For this review, take the finished solid that the model builds, in its own axes (mm). A direction names the side the tool comes from. Coordinates: 2 decimals unless noted, no trailing zeros. Loops run counter-clockwise (first coordinate to the right, second up) from the corner with the lowest first, then second, coordinate; pieces in that order, holes last. Notation, with made-up numbers: (71, 69.5) -> (98, 69.5) arc R27 cw to (98, 85.5) -> close; hole circle Ø10 at (-32, 47.25). An arc over 180 degrees is marked (long way). Use a Markdown table: item, result.
Autodesk Inventor part; units mm, degrees
ref_plane "Work Plane1" through (3.5, 0, 0) normal (1, 0, 0) x (0, 1, 0)
ref_plane "XZ Plane" through (0, 0, 0) normal (0, 1, 0) x (-1, 0, 0)
ref_plane "XY Plane" through (0, 0, 0) normal (0, 0, 1) x (1, 0, 0)
sketch "Sketch1" plane through (0, 0, 0) normal (0, 1, 0) x (-1, 0, 0)
  circle A0 centre (0, 0) radius 2.2
  circle A1 centre (0, 0) radius 4.5
  dimension "d0" = 4.4
  dimension "d1" = 9
extrude "Extrusion1" add sketch "Sketch1" along normal blind 15 contours A0 | A1
sketch "Sketch2" plane through (0, 15, 0) normal (0, 1, 0) x (1, 0, 0)
  circle A0 centre (0, 0) radius 2.2
  dimension "d4" = 4.4
ref_plane "Work Plane1" through (3.5, 0, 0) normal (1, 0, 0) x (0, 1, 0)
sketch "Sketch3" plane through (3.5, 0, 0) normal (1, 0, 0) x (0, 1, 0)
  line L0 (0, 0) -> (7.5, 0)
  circle A0 centre (7.5, 0) radius 5.5
  dimension "d13" = 7.5
  dimension "d15" = 11
extrude "Extrusion2" add sketch "Sketch3" along normal mid plane 30
sketch "Sketch6" plane through (-11.5, 0, 0) normal (-1, 0, 0) x (0, 0, 1)
  circle A0 centre (0, 7.5) radius 5.5
  arc A1 (0, 11) -> (0, 4) centre (0, 7.5) ccw
  line L0 (0, 2) -> (0, 13)
  line L1 (0, 11) -> (0, 4)
  point P0 (0, 0)
sketch "Sketch7" plane through (18.5, 7.5, 0) normal (1, 0, 0) x (0, 0, -1)
  point P0 (0, -7.5)
hole "Hole4" at (0, 15, 0) direction (0, -1, 0) diameter 4.5 depth 20
sketch "Sketch8" plane through (18.5, 7.5, 0) normal (1, 0, 0) x (0, 0, -1)
  circle A0 centre (0, 0) radius 3
  point P0 (0, -7.5)
  dimension "d44" = 6
hole "Hole5" at (18.5, 7.5, 0) direction (-1, 0, 0) diameter 6 depth 15
properties part number "codo"
(1) Mouldability with a two-part tool opening along Y and no side actions: class faces 1 (the face through (-2, 15, -2)), 2 (the face through (10.895, 4.526, 0.391)), 3 (the face through (3.5, 7, 0)), 4 (the face through (18.5, 10, -2)) as pulls with the +Y half, pulls with the -Y half, needs draft (parallel to the pull), parting line crosses it, or undercut.
Found:
| item | result |
|---|---|
| face 1 | pulls with the +Y half |
| face 2 | undercut |
| face 3 | undercut |
| face 4 | needs draft |
(2) Take a section at C-C on y = 7.5. Write out the cut boundary in (x, z).
Found:
| item | result |
|---|---|
| outline | (-11.5, -5.5) -> (18.5, -5.5) -> (18.5, -3) -> (3.5, -3) -> (3.5, 3) -> (18.5, 3) -> (18.5, 5.5) -> (-11.5, 5.5) -> close; hole circle Ø4.5 at (0, 0) |
(3) For faces 5 (the face through (3.71, 6.784, 5.453)), 6 (the face through (0.98, 13.28, 4.39)), 7 (the face through (-2.08, 1.66, 3.99)), list the 3-axis set-ups (+Z, -Z, +X, -X, +Y, -Y) from which the entire face can be reached by the end or side of a thin tool; tool diameter is ignored.
Found:
| item | result |
|---|---|
| face 5 | none |
| face 6 | +Y |
| face 7 | -Y |
(4) Take a section at D-D on x = -9.5. Write out the cut boundary in (y, z).
Found:
| item | result |
|---|---|
| outline | circle Ø11 at (7.5, 0) |
(5) Take a section at A-A on z = 0. Write out the cut boundary in (x, y), plus the area to 4 significant figures.
Found:
| item | result |
|---|---|
| outline | (-11.5, 2) -> (-4.5, 2) -> (-4.5, 0) -> (-2.25, 0) -> (-2.25, 15) -> (-4.5, 15) -> (-4.5, 13) -> (-11.5, 13) -> close; (2.25, 0) -> (4.5, 0) -> (4.5, 2) -> (18.5, 2) -> (18.5, 4.5) -> (3.5, 4.5) -> (3.5, 10.5) -> (18.5, 10.5) -> (18.5, 13) -> (4.5, 13) -> (4.5, 15) -> (2.25, 15) -> close |
| area | 208.5 mm^2 |
(6) For pin 1 Ø2 at (x, z) = (-8.5, 2.5) entering from -Y; pin 2 Ø1.5 at (x, y) = (-3, 1.5) entering from +Z; pin 3 Ø4 at (x, z) = (-1, 0) entering from -Y; pin 4 Ø2 at (x, z) = (7, 2.5) entering from +Y, all flat-tipped, find the tip position at first contact; note any pin that passes through.
Found:
| item | result |
|---|---|
| pin 1 | stops at y = 2.21 |
| pin 2 | stops at z = 3.9 |
| pin 3 | stops at y = 0 |
| pin 4 | stops at y = 12.79 |
(7) For line 1 along X through (y, z) = (14.25, 0); line 2 along Y through (x, z) = (12.5, 0); line 3 along X through (y, z) = (6.75, 0), list the stretches that pass through material, from the lowest coordinate up.
Found:
| item | result |
|---|---|
| line 1 | x = -4.5 to -2.25, 2.25 to 4.5 |
| line 2 | y = 2 to 4.5, 10.5 to 13 |
| line 3 | x = -11.5 to -2.25, 2.25 to 3.5 |
(8) Take a section at B-B on x = 0. Write out the cut boundary in (y, z).
Found:
| item | result |
|---|---|
| outline | (0, -4.5) -> (4.34, -4.5) arc R5.5 ccw to (10.66, -4.5) -> (15, -4.5) -> (15, -2.25) -> (0, -2.25) -> close; (0, 2.25) -> (15, 2.25) -> (15, 4.5) -> (10.66, 4.5) arc R5.5 ccw to (4.34, 4.5) -> (0, 4.5) -> close |
